```python
from build123d import *

# Parameters (mm, degrees)
SKETCH_1_R          = 1.7
SKETCH_1_R_2        = 7.046714779
EXTRUDE_2_DEPTH     = 8
SKETCH_2_W          = 10
SKETCH_2_H          = 56
EXTRUDE_3_DEPTH     = 58
SKETCH_3_R          = 1.45
SKETCH_3_R_2        = 10
CUT_EXTRUDE_1_DEPTH = 22
SKETCH_5_W          = 10
SKETCH_5_H          = 20.367119739
CUT_EXTRUDE_3_DEPTH = 18
CHAMFER_1_SIZE      = 5
FILLET_1_R          = 30
SKETCH_6_R          = 3.2
CUT_EXTRUDE_4_DEPTH = 4
SKETCH_7_R          = 3.2
CUT_EXTRUDE_5_DEPTH = 3
EXTRUDE_4_DEPTH     = 4
SKETCH_9_R          = 28
CUT_EXTRUDE_6_DEPTH = 10
CHAMFER_2_SIZE      = 4


# Some blends are built 0.0001 mm under size
with BuildPart() as part:
    # 草图1 → 凸台-拉伸2 (new body)
    with BuildSketch(Plane(origin=(0, 0, 0), x_dir=(1, 0, 0), z_dir=(0, 1, 0))):
        with BuildLine():
            Line((-23, 28), (-33, 28))
            Line((-33, 28), (-33, -28))
            Line((-33, -28), (-23, -28))
            Line((-23, -28), (0, -28))
            ThreePointArc((0, -28), (28, 0), (0, 28))
            Line((0, 28), (-23, 28))
        make_face()
        with Locations(Location((0, 13.5, 0), (0, 0, 270))):
            Circle(SKETCH_1_R, mode=Mode.SUBTRACT)
        with Locations(Location((11.691342951, -6.75, 0), (0, 0, 270))):
            Circle(SKETCH_1_R, mode=Mode.SUBTRACT)
        with Locations(Location((-11.691342951, -6.75, 0), (0, 0, 270))):
            Circle(SKETCH_1_R, mode=Mode.SUBTRACT)
        with Locations(Location((0, 0, 0), (0, 0, 270))):
            Circle(SKETCH_1_R_2, mode=Mode.SUBTRACT)
    extrude(amount=EXTRUDE_2_DEPTH)

    # 草图2 → 凸台-拉伸3 (add)
    with BuildSketch(Plane(origin=(0, 8, 0), x_dir=(1, 0, 0), z_dir=(0, 1, 0))):
        with Locations((-28, 0)):
            Rectangle(SKETCH_2_W, SKETCH_2_H)
    extrude(amount=EXTRUDE_3_DEPTH)

    # 草图3 → 切除-拉伸1 (cut)
    with BuildSketch(Plane(origin=(-23, 0, 0), x_dir=(0, 0, -1), z_dir=(1, 0, 0))):
        with Locations((0, 55.2)):
            Circle(SKETCH_3_R)
        with Locations((19, 36.2)):
            Circle(SKETCH_3_R)
        with Locations((0, 17.2)):
            Circle(SKETCH_3_R)
        with Locations((-19, 36.2)):
            Circle(SKETCH_3_R)
        with Locations((0, 36.2)):
            Circle(SKETCH_3_R_2)
    extrude(amount=-CUT_EXTRUDE_1_DEPTH, mode=Mode.SUBTRACT)

    # 草图5 → 切除-拉伸3 (cut)
    with BuildSketch(Plane(origin=(0, 8, 0), x_dir=(1, 0, 0), z_dir=(0, 1, 0))):
        with Locations((-18, 33.18355987)):
            Rectangle(SKETCH_5_W, SKETCH_5_H)
        with Locations((-18, -33.18355987)):
            Rectangle(SKETCH_5_W, SKETCH_5_H)
    extrude(amount=-CUT_EXTRUDE_3_DEPTH, mode=Mode.SUBTRACT)

    # 倒角1
    chamfer_1_edges = [part.edges().sort_by_distance(p)[0] for p in [
        (-23, 33, 28),
        (-23, 33, -28),
        (-13, 4, -28),
        (-13, 4, 28),
    ]]
    chamfer(chamfer_1_edges, length=CHAMFER_1_SIZE - 0.0001)  # a hair under: the kernel refuses the full size

    # 圆角1
    # the kernel refuses this fillet: 30 mm, written as the material it takes off along each edge
    with BuildSketch(Plane(origin=(-108, 66, -28), x_dir=(0, -1, 0), z_dir=(1, 0, 0)), Plane(origin=(47.0001, 66, 28), x_dir=(0, -1, 0), z_dir=(-1, 0, 0))) as fillet_1_piece_1:
        with BuildLine():
            CenterArc((FILLET_1_R, -FILLET_1_R), FILLET_1_R, 90, 90)
            Line((0, -FILLET_1_R), (0, 0))
            Line((0, 0), (FILLET_1_R, 0))
        make_face()
    extrude(amount=155.0001, mode=Mode.SUBTRACT)

    # 草图6 → 切除-拉伸4 (cut)
    with BuildSketch(Plane.ZY.offset(33)):
        with Locations((-19, 36.2)):
            Circle(SKETCH_6_R)
        with Locations((0, 55.2)):
            Circle(SKETCH_6_R)
        with Locations((19, 36.2)):
            Circle(SKETCH_6_R)
        with Locations((0, 17.2)):
            Circle(SKETCH_6_R)
    extrude(amount=-CUT_EXTRUDE_4_DEPTH, mode=Mode.SUBTRACT)

    # 草图7 → 切除-拉伸5 (cut)
    with BuildSketch(Plane(origin=(0, 8, 0), x_dir=(1, 0, 0), z_dir=(0, 1, 0))):
        with Locations(Location((0, 13.5, 0), (0, 0, 270))):
            Circle(SKETCH_7_R)
        with Locations(Location((11.691342951, -6.75, 0), (0, 0, 270))):
            Circle(SKETCH_7_R)
        with Locations(Location((-11.691342951, -6.75, 0), (0, 0, 270))):
            Circle(SKETCH_7_R)
    extrude(amount=-CUT_EXTRUDE_5_DEPTH, mode=Mode.SUBTRACT)

    # 草图8 → 凸台-拉伸4 (add)
    with BuildSketch(Plane(origin=(0, 8, 0), x_dir=(1, 0, 0), z_dir=(0, 1, 0))):
        with BuildLine():
            Line((17, -22.248595461), (17, 22.248595461))
            ThreePointArc((17, 22.248595461), (18.01962739, 21.4311229), (19, 20.566963801))
            Line((19, 20.566963801), (19, -20.566963801))
            ThreePointArc((19, -20.566963801), (18.01962739, -21.4311229), (17, -22.248595461))
        make_face()
    extrude(amount=EXTRUDE_4_DEPTH)

    # 草图9 → 切除-拉伸6 (cut)
    with BuildSketch(Plane(origin=(19, 0, 0), x_dir=(0, 0, -1), z_dir=(1, 0, 0))):
        with Locations((0, 36.2)):
            Circle(SKETCH_9_R)
    extrude(amount=-CUT_EXTRUDE_6_DEPTH, mode=Mode.SUBTRACT)

    # 倒角2
    # the kernel refuses this chamfer: 4 mm, written as the material it takes off along each edge
    with BuildSketch(Plane(origin=(0, 8, 28), x_dir=(0, 0.027495876610586487, -0.9996219169112968), z_dir=(-1, 0, 0))) as chamfer_2_piece_1:
        Polygon((CHAMFER_2_SIZE * 0.999621916911, CHAMFER_2_SIZE * 0.0274958766106), (-CHAMFER_2_SIZE * 0.0274958766106, CHAMFER_2_SIZE * 0.999621916911), (0, 0), align=None)
    extrude(amount=18.286831952, mode=Mode.SUBTRACT)
    with BuildSketch(Plane(origin=(0, 8, 0), x_dir=(0.369313229341893, 0, 0.9293049761155173), z_dir=(-0.9293049761155173, 0, 0.369313229341893))) as chamfer_2_piece_2_section:
        Polygon((28, -CHAMFER_2_SIZE), (28 - CHAMFER_2_SIZE, 0), (28, 0), align=None)
    chamfer_2_piece_2 = revolve(axis=Axis((0, 8, 0), (0, 1, 0)), revolution_arc=136.653462803, mode=Mode.PRIVATE)
    chamfer_2_piece_2 = split(chamfer_2_piece_2, bisect_by=Plane(origin=(17, 6.694433411, 22.783727906), z_dir=(-1, 0, 0)), keep=Keep.TOP, mode=Mode.PRIVATE)
    add(chamfer_2_piece_2, mode=Mode.SUBTRACT)
    with BuildSketch(Plane(origin=(0, 8, 0), x_dir=(0.369313229341893, 0, 0.9293049761155173), z_dir=(-0.9293049761155173, 0, 0.369313229341893))) as chamfer_2_piece_3_section:
        Polygon((28, -CHAMFER_2_SIZE), (28 - CHAMFER_2_SIZE, 0), (28, 0), align=None)
    chamfer_2_piece_3 = revolve(axis=Axis((0, 8, 0), (0, 1, 0)), revolution_arc=136.653462803, mode=Mode.PRIVATE)
    chamfer_2_piece_3 = split(chamfer_2_piece_3, bisect_by=Plane(origin=(19, 6.048939882, 0), z_dir=(1, 0, 0)), keep=Keep.TOP, mode=Mode.PRIVATE)
    add(chamfer_2_piece_3, mode=Mode.SUBTRACT)
    with BuildSketch(Plane(origin=(0, 8, 0), x_dir=(0.8520392640465919, 0, -0.5234778815985848), z_dir=(0.5234778815985848, 0, 0.8520392640465919))) as chamfer_2_piece_4_section:
        Polygon((28, -CHAMFER_2_SIZE), (28 - CHAMFER_2_SIZE, 0), (28, 0), align=None)
    chamfer_2_piece_4 = revolve(axis=Axis((0, 8, 0), (0, 1, 0)), revolution_arc=58.434168598, mode=Mode.PRIVATE)
    chamfer_2_piece_4 = split(chamfer_2_piece_4, bisect_by=Plane(origin=(19, 6.574014783, -16.582020982), z_dir=(1, 0, 0)), keep=Keep.TOP, mode=Mode.PRIVATE)
    add(chamfer_2_piece_4, mode=Mode.SUBTRACT)
    with BuildSketch(Plane(origin=(0, 8, 0), x_dir=(0.8520392640465919, 0, -0.5234778815985848), z_dir=(0.5234778815985848, 0, 0.8520392640465919))) as chamfer_2_piece_5_section:
        Polygon((28, -CHAMFER_2_SIZE), (28 - CHAMFER_2_SIZE, 0), (28, 0), align=None)
    chamfer_2_piece_5 = revolve(axis=Axis((0, 8, 0), (0, 1, 0)), revolution_arc=58.434168598, mode=Mode.PRIVATE)
    chamfer_2_piece_5 = split(chamfer_2_piece_5, bisect_by=Plane(origin=(17, 6.670131388, -24.579888545), z_dir=(-1, 0, 0)), keep=Keep.TOP, mode=Mode.PRIVATE)
    add(chamfer_2_piece_5, mode=Mode.SUBTRACT)
    with BuildSketch(Plane(origin=(0, 8, 0), x_dir=(0, 0, 1), z_dir=(-1, 0, 0))) as chamfer_2_piece_6_section:
        Polygon((28, -CHAMFER_2_SIZE), (28 - CHAMFER_2_SIZE, 0), (28, 0), align=None)
    chamfer_2_piece_6 = revolve(axis=Axis((0, 8, 0), (0, 1, 0)), revolution_arc=58.434168598, mode=Mode.PRIVATE)
    chamfer_2_piece_6 = split(chamfer_2_piece_6, bisect_by=Plane(origin=(17, 6.670131388, 24.579888545), z_dir=(-1, 0, 0)), keep=Keep.TOP, mode=Mode.PRIVATE)
    add(chamfer_2_piece_6, mode=Mode.SUBTRACT)
    with BuildSketch(Plane(origin=(0, 8, 0), x_dir=(0, 0, 1), z_dir=(-1, 0, 0))) as chamfer_2_piece_7_section:
        Polygon((28, -CHAMFER_2_SIZE), (28 - CHAMFER_2_SIZE, 0), (28, 0), align=None)
    chamfer_2_piece_7 = revolve(axis=Axis((0, 8, 0), (0, 1, 0)), revolution_arc=58.434168598, mode=Mode.PRIVATE)
    chamfer_2_piece_7 = split(chamfer_2_piece_7, bisect_by=Plane(origin=(19, 6.574014783, 16.582020982), z_dir=(1, 0, 0)), keep=Keep.TOP, mode=Mode.PRIVATE)
    add(chamfer_2_piece_7, mode=Mode.SUBTRACT)
    with BuildSketch(Plane(origin=(-18.286831952, 8, -28), x_dir=(0, -0.9996219169112968, -0.027495876610586487), z_dir=(1, 0, 0))) as chamfer_2_piece_8:
        Polygon((CHAMFER_2_SIZE * 0.999621916911, -CHAMFER_2_SIZE * 0.0274958766106), (-CHAMFER_2_SIZE * 0.0274958766106, -CHAMFER_2_SIZE * 0.999621916911), (0, 0), align=None)
    extrude(amount=18.286831952, mode=Mode.SUBTRACT)


solid = part.part
```
Source: CAD feature listing. Evaluate the final solid. Frame: model axes, mm. A direction names the side the tool comes from. Give positions to 0.01 mm unless a question says otherwise; leave off trailing zeros. Loops run counter-clockwise (first coordinate to the right, second up) from the corner with the lowest first, then second, coordinate; pieces in that order, holes last. Notation, with made-up numbers: (24, 32.25) -> (74, 32.25) arc R10 ccw to (74, 48.25) -> close; hole circle Ø2 at (2, -23). An arc over 180 degrees is marked (long way). Use a Markdown table: item, result. Add a question column.
(1) Section query D-D (y = 51). Output: boundary loops of the cut face in (x, z).
(2) Access query for faces 1 (the face through (-26, 27, -26)), 2 (the face through (-29, 38, 19)), 3 (the face through (-10.006, 2.465, 6.529)), 4 (the face through (10, 5, 8)). Directions: +Z, -Z, +X, -X, +Y, -Y. A direction counts if a zero-diameter tool reaches every point of the face in a straight line with its end or side. Return the directions, or none.
(3) Section query A-A (x = -5.5). Output: boundary loops of the cut face in (y, z), then the cut area to 3 significant figures.
(4) Section query B-B (y = 9.5). Output: boundary loops of the cut face in (x, z), then the cut area to 3 significant figures.
(5) Ray query, line 1 (Z direction, x = -24, y = 36); line 2 (Y direction, x = -7, z = -19); line 3 (Y direction, x = -26.5, z = 19). Return the intervals inside material, ascending.
(6) First-contact query: pin 1 Ø4 at (y, z) = (36.2, 19) entering from -X; pin 2 Ø1 at (x, z) = (19, -5) entering from +Y; pin 3 Ø2.5 at (y, z) = (8.5, -1) entering from +X; pin 4 Ø1.9 at (x, z) = (-0.5, -13) entering from +Y. Flat tips, straight axial feed; report the tip coordinate or a pass-through.
(7) Section query C-C (x = -27). Output: boundary loops of the cut face in (y, z).
(8) Pull-direction query (Y, two-part tool) for faces 5 (the face through (-33, 25, 0)), 6 (the face through (-27.93, 56.262, 20.123)), 7 (the face through (-25.958, 18.638, 0.189)), 8 (the face through (-10, 0, 0)); classes: +Y half, -Y half, draft (parallel to the pull), parting line (faces both ways), or undercut.
Checked values:
| question | item | result |
|---|---|---|
| 1 | outline | (-33, -23.98) -> (-23.98, -23.98) -> (-23, -23) -> (-23, 23) -> (-23.98, 23.98) -> (-33, 23.98) -> close |
| 2 | face 1 | -Z, +Y, -Y |
| 2 | face 2 | -X |
| 2 | face 3 | +Y, -Y |
| 2 | face 4 | +Y |
| 3 | outline | (0, -28) -> (4, -28) -> (8, -24) -> (8, -4.41) -> (0, -4.41) -> close; (0, 4.41) -> (8, 4.41) -> (8, 24) -> (4, 28) -> (0, 28) -> close |
| 3 | area | 362 mm^2 |
| 4 | outline | (-33, -28) -> (-28, -28) -> (-23, -23) -> (-23, 23) -> (-28, 28) -> (-33, 28) -> close; (17, -22.25) arc R28 ccw to (19, -20.57) -> (19, -8.43) -> (17, -8.43) -> close; (17, 8.43) -> (19, 8.43) -> (19, 20.57) arc R28 ccw to (17, 22.25) -> close |
| 4 | area | 587 mm^2 |
| 5 | line 1 | -24 to -20.44, -17.56 to -10, 10 to 17.56, 20.44 to 24 |
| 5 | line 2 | 0 to 8 |
| 5 | line 3 | 0 to 34.75, 37.65 to 57.42 |
| 6 | pin 1 | x = -29 |
| 6 | pin 2 | y = 8.75 |
| 6 | pin 3 | x = 24.73 |
| 6 | pin 4 | through |
| 7 | outline | (0, -27) -> (43.68, -27) arc R30 ccw to (65.93, 0) arc R30 ccw to (43.68, 27) -> (0, 27) -> close; hole circle Ø2.9 at (17.2, 0); hole circle Ø20 at (36.2, 0); hole circle Ø2.9 at (36.2, -19); hole circle Ø2.9 at (36.2, 19); hole circle Ø2.9 at (55.2, 0) |
| 8 | face 5 | draft |
| 8 | face 6 | +Y half |
| 8 | face 7 | undercut |
| 8 | face 8 | -Y half |
